Check sheet for the modelled part. Datum: model origin and axes. Units: mm. Face numbers are marked on the shaded views. A direction names the side the tool comes from. Give positions to 0.01 mm unless a question says otherwise; leave off trailing zeros. Loops run counter-clockwise (first coordinate to the right, second up) from the corner with the lowest first, then second, coordinate; pieces in that order, holes last.
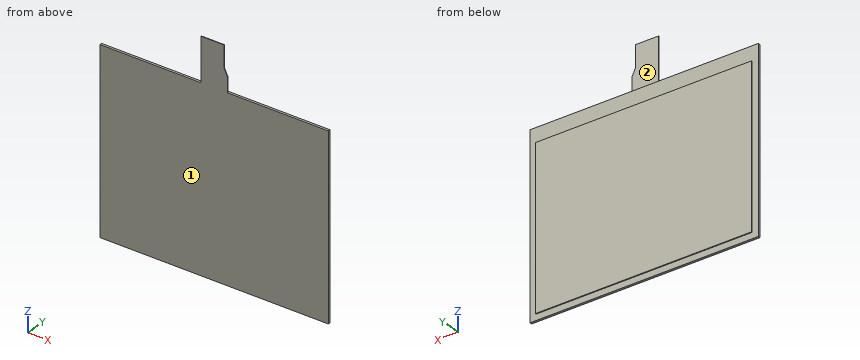
```python
from build123d import *

# Parameters (mm, degrees)
SKETCH1_W           = 125.5
SKETCH1_H           = 99.6
BOSS_EXTRUDE1_DEPTH = 1.25
SKETCH2_W           = 118.78
SKETCH2_H           = 88.22
BOSS_EXTRUDE2_DEPTH = 0.55
BOSS_EXTRUDE3_DEPTH = 0.315


with BuildPart() as part:
    # Sketch1 → Boss-Extrude1 (new body)
    with BuildSketch(Plane(origin=(0, 0, 0), x_dir=(1, 0, 0), z_dir=(0, 1, 0))):
        with Locations((62.75, -49.8)):
            Rectangle(SKETCH1_W, SKETCH1_H)
    extrude(amount=BOSS_EXTRUDE1_DEPTH)

    # Sketch2 → Boss-Extrude2 (add)
    with BuildSketch(Plane(origin=(0, 1.25, 0), x_dir=(1, 0, 0), z_dir=(0, 1, 0))):
        with Locations((62.75, -47.41)):
            Rectangle(SKETCH2_W, SKETCH2_H)
    extrude(amount=BOSS_EXTRUDE2_DEPTH)

    # Sketch3 → Boss-Extrude3 (add)
    with BuildSketch(Plane.XZ):
        Polygon((55.57, 99.6), (70.03, 99.6), (70.03, 107.87048089), (68.07, 112.011323717), (68.07, 123.6), (55.57, 123.6), align=None)
    extrude(amount=-BOSS_EXTRUDE3_DEPTH)


solid = part.part
```
(1) Access from +Z, -Z, +X, -X, +Y, -Y to the whole of each face (thin tool, end or side, straight path). Record for the marked faces 1 and 2.
(2) Section check B-B on x = 81. Record the boundary of the cut face in (y, z).
(3) Gauge pin test, flat end, axial feed: pin 1 Ø11.5 at (x, z) = (63.5, 107.5) entering from +Y (3 decimals). Record the tip position at first contact, or that the pin passes through.
(4) Material ranges on line 1 (X direction, y = 1.3, z = 46.5); line 2 (Z direction, x = 97.5, y = 0.15); line 3 (Z direction, x = 101.5, y = 1.55), recorded low to high.
(5) Section check C-C on z = 116.5. Record the boundary of the cut face in (x, y) (3 decimals).
(6) Section check A-A on z = 35. Record the boundary of the cut face in (x, y).
Computed values:
1. face 1: +Z, -Z, +X, -X, -Y
1. face 2: +Z, +X, -X, +Y
2. outline: (0, 0) - (1.25, 0) - (1.25, 3.3) - (1.8, 3.3) - (1.8, 91.52) - (1.25, 91.52) - (1.25, 99.6) - (0, 99.6) - close
3. pin 1: stops at y = 0.315
4. line 1: x = 3.36 to 122.14
4. line 2: z = 0 to 99.6
4. line 3: z = 3.3 to 91.52
5. outline: (55.57, 0) - (68.07, 0) - (68.07, 0.315) - (55.57, 0.315) - close
6. outline: (0, 0) - (125.5, 0) - (125.5, 1.25) - (122.14, 1.25) - (122.14, 1.8) - (3.36, 1.8) - (3.36, 1.25) - (0, 1.25) - close
